Verification items for the finished model (mm, model axes). Round coordinates to 2 decimals unless told otherwise and drop trailing zeros. Order: outer loops, then holes, each group sorted by start corner. A loop starts at its lowest first (then second) coordinate and runs counter-clockwise, first axis right, second up. Notation, with made-up numbers: M 17.25,38.25 L 39.25,38.25 A23 cw 39.25,72.25 Z; hole C 30.5,38 d1. An arc over 180 degrees is marked long. One line per item, written item: value. Start each with the question number.
from build123d import *

# Parameters (mm, degrees)
F0_W     = 60
F0_H     = 20
F1_DEPTH = 40
F3_R     = 4
F4_D     = 6
F5_W     = 10
F5_H     = 10
F6_DEPTH = 508


with BuildPart() as f1:
    # F0 (on Front) → F1 (new body)
    with BuildSketch(Plane.XZ):
        with Locations((30, -10)):
            Rectangle(F0_W, F0_H)
    extrude(amount=F1_DEPTH)

    # F3
    f3_edges = [f1.edges().sort_by_distance(p)[0] for p in [
        (60, 0, -10),
        (0, -20, -20),
        (0, 0, -10),
        (0, -20, 0),
        (0, -40, -10),
        (60, -20, -20),
        (60, -40, -10),
        (60, -20, 0),
        (30, -40, 0),
        (30, -40, -20),
        (30, 0, -20),
        (30, 0, 0),
    ]]
    fillet(f3_edges, radius=F3_R)

    # F4 (through all)
    with Locations(Plane.XY):
        with Locations((40, -20)):
            Hole(F4_D / 2)

    # F5 (on face) → F6 (join)
    with BuildSketch(Plane(origin=(0, 0, -20), x_dir=(1, 0, 0), z_dir=(0, 0, -1))):
        with Locations((25, 20)):
            Rectangle(F5_W, F5_H)
    extrude(amount=-F6_DEPTH)


solid = f1.part
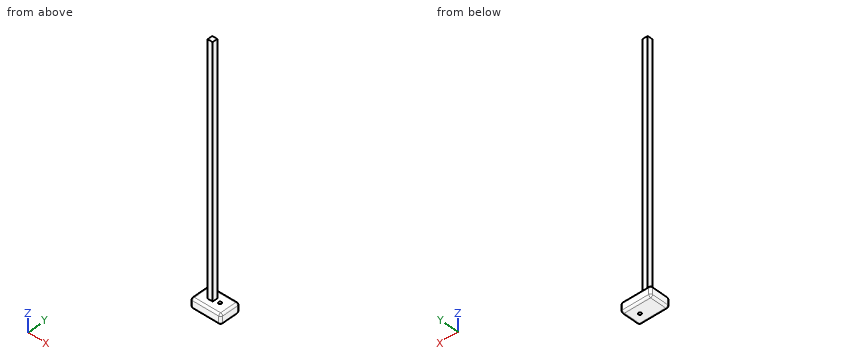
1. Depth check by flat-ended pin: pin 1 (10 mm diameter, centred on y = -16, z = 307.5, fed in from -X); pin 2 (11 mm diameter, centred on x = 26.5, z = 261, fed in from -Y); pin 3 (3.5 mm diameter, centred on x = 40, y = -20, fed in from -Z); pin 4 (1 mm diameter, centred on x = 12.5, y = -11, fed in from +Z). Enter the tip coordinate at first touch or a pass-through.
2. Section check A-A (x = 50). Record the cut outline in (y, z).
3. Scan lines: line 1 along Y through (x, z) = (40, -13); line 2 along Z through (x, y) = (3.5, -7.5); line 3 along Y through (x, z) = (26, 452.5). Record each from-to range of solid material in increasing order.
4. Section check B-B (z = 226). Record the cut outline in (x, y), and give its area (3 significant figures).
Geometry check:
1. pin 1: stops at x = 20
1. pin 2: stops at y = -25
1. pin 3: passes through
1. pin 4: stops at z = 0
2. outline: M -40,-16 A4 ccw -36,-20 L -4,-20 A4 ccw 0,-16 L 0,-4 A4 ccw -4,0 L -36,0 A4 ccw -40,-4 Z
3. line 1: y = -40 to -23, -17 to 0
3. line 2: z = -19.97 to -0.03
3. line 3: y = -25 to -15
4. outline: M 20,-25 L 30,-25 L 30,-15 L 20,-15 Z
4. area: 100 mm²
